Could you check a few things on this drawing? It's one solid part, dimensions in mm from its lowest x, y, z. A direction names the side the tool comes from. Coordinates: 2 decimals unless noted, no trailing zeros. Loops run counter-clockwise (first coordinate to the right, second up) from the corner with the lowest first, then second, coordinate; pieces in that order, holes last.
1) Thinking about a two-plate mould opening in Z: for the marked faces 4, 5 and 6, which applies, released by +Z, released by -Z, zero draft, split by the parting line, or undercut?
2) Will these pins go through, and if not, where does the flat tip stop? P1, Ø0.7, axis at x = 7, z = 5.5, coming from the -Y side; P2, Ø1, axis at x = 3, z = 6.5, coming from the +Y side; P3, Ø1.6, axis at x = 9.5, z = 2.5, coming from the -Y side.
3) For the marked faces 1, 2 and 3, which set-ups out of +Z, -Z, +X, -X, +Y, -Y let a thin tool reach every point of the face, with its end or its side?
4) Imagine slicing it at A-A on y = 4. Please give me the cut outline in (x, z), plus the area to 3 significant figures.
5) If I drill on line 1 along Z through (x, y) = (3.6, 4); line 2 along Z through (x, y) = (5.25, 4); line 3 along X through (y, z) = (5.5, 5.5), over which ranges is the centre line in solid material (lowest first)?
6) Imagine slicing it at D-D on z = 1.25. Please give me the cut outline in (x, y).
7) Imagine slicing it at C-C on x = 10.25. Please give me the cut outline in (y, z).
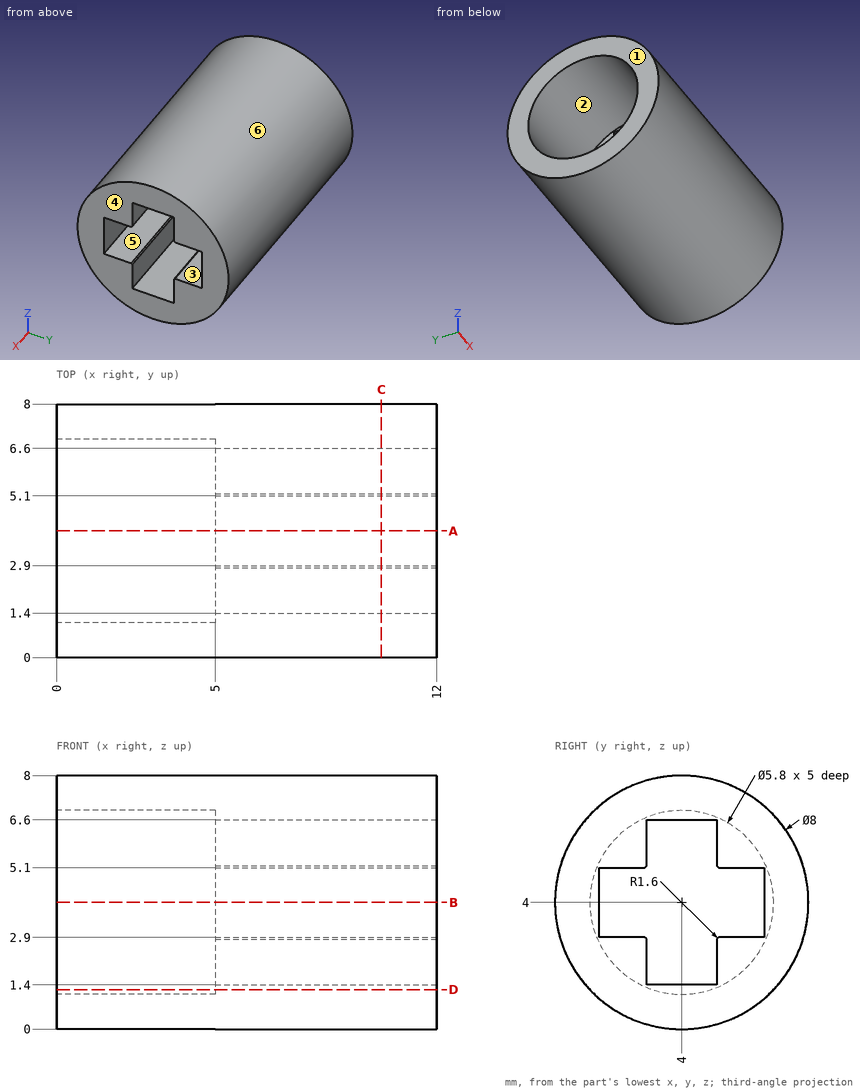
Filled in:
1. face 4: zero draft
1. face 5: undercut
1. face 6: split by the parting line
2. P1: stops at y = 0.17
2. P2: stops at y = 7.46
2. P3: stops at y = 0.06
3. face 1: +Z, -Z, -X, +Y, -Y
3. face 2: -X
3. face 3: +X, -X
4. outline: (0, 0) - (12, 0) - (12, 1.4) - (5, 1.4) - (5, 1.1) - (0, 1.1) - close; (0, 6.9) - (5, 6.9) - (5, 6.6) - (12, 6.6) - (12, 8) - (0, 8) - close
4. area: 30.6 mm2
5. line 1: z = 0 to 1.1, 6.9 to 8
5. line 2: z = 0 to 1.4, 6.6 to 8
5. line 3: x = 5 to 12
6. outline: (0, 1.1) - (12, 1.1) - (12, 6.9) - (0, 6.9) - (0, 4.92) - (5, 4.92) - (5, 3.08) - (0, 3.08) - close
7. outline: circle Ø8 at (4, 4); hole (1.4, 2.9) - (2.84, 2.9) arc R1.6 ccw to (2.9, 2.84) - (2.9, 1.4) - (5.1, 1.4) - (5.1, 2.84) arc R1.6 ccw to (5.16, 2.9) - (6.6, 2.9) - (6.6, 5.1) - (5.16, 5.1) arc R1.6 ccw to (5.1, 5.16) - (5.1, 6.6) - (2.9, 6.6) - (2.9, 5.16) arc R1.6 ccw to (2.84, 5.1) - (1.4, 5.1) - close
